Check sheet for the modelled part. Datum: model origin and axes. Units: mm. A direction names the side the tool comes from. Round coordinates to 2 decimals unless told otherwise and drop trailing zeros. Order: outer loops, then holes, each group sorted by start corner. A loop starts at its lowest first (then second) coordinate and runs counter-clockwise, first axis right, second up.
```python
from build123d import *

# Parameters (mm, degrees)
F2_R      = 31.4610783887
F2_R_2    = 24.995840748
F3_DEPTH  = 33.02
F4_R      = 38.1
F4_R_2    = 31.4610783887
F4_R_3    = 24.995840748
F5_DEPTH  = 35.56
F6_SIZE   = 12.7
F8_W      = 7.62
F8_H      = 11.43
F9_DEPTH  = 15.7618920784
F10_SIZE  = 5.08
F11_R     = 3.175
F12_DEPTH = 5.08
F13_R     = 3.175
F14_DEPTH = 5.08


with BuildPart() as f3:
    # F2 (on offset) → F3 (new body)
    with BuildSketch(Plane.XY.offset(-98.8788958639)):
        Circle(F2_R)
        Circle(F2_R_2, mode=Mode.SUBTRACT)
    extrude(amount=-F3_DEPTH)

    # F4 (on face) → F5 (join)
    with BuildSketch(Plane(origin=(0, 0, -131.8988958639), x_dir=(1, 0, 0), z_dir=(0, 0, -1))):
        Circle(F4_R)
        Circle(F4_R_2, mode=Mode.SUBTRACT)
        Circle(F4_R_2)
        Circle(F4_R_3, mode=Mode.SUBTRACT)
        Circle(F4_R_3)
    extrude(amount=F5_DEPTH)

    # F6
    f6_edges = [f3.edges().sort_by_distance(p)[0] for p in [
        (-38.1, 0, -167.458896),
    ]]
    chamfer(f6_edges, length=F6_SIZE)

    # F8 (on face) → F9 (join)
    with BuildSketch(Plane(origin=(0, 0, -167.4588958639), x_dir=(1, 0, 0), z_dir=(0, 0, -1))):
        with Locations((0, 29.3979875922)):
            Rectangle(F8_W, F8_H)
        Polygon((-12.3045016564, 20.5912418344), (-19.6515640351, 29.3471298192), (-25.4888226916, 24.4490882334), (-18.1417603129, 15.6932002486), align=None)
        Polygon((-22.6615902384, 7.8646251761), (-33.9179428553, 9.8494238468), (-35.2411419691, 2.3451887689), (-23.9847893522, 0.3603900981), align=None)
        Polygon((-22.4150688924, -8.5419370077), (-32.3137392576, -14.2569370077), (-28.5037392576, -20.8560505845), (-18.6050688924, -15.1410505845), align=None)
        Polygon((-11.6802876959, -20.9516319325), (-15.5895779341, -31.6923185881), (-8.4291201637, -34.2985120802), (-4.5198299255, -23.5578254246), align=None)
        Polygon((4.5198299255, -23.5578254246), (8.4291201637, -34.2985120802), (15.5895779341, -31.6923185881), (11.6802876959, -20.9516319325), align=None)
        Polygon((18.6050688924, -15.1410505845), (28.5037392576, -20.8560505845), (32.3137392576, -14.2569370077), (22.4150688924, -8.5419370077), align=None)
        Polygon((23.9847893522, 0.3603900981), (35.2411419691, 2.3451887689), (33.9179428553, 9.8494238468), (22.6615902384, 7.8646251761), align=None)
        Polygon((18.1417603129, 15.6932002486), (25.4888226916, 24.4490882334), (19.6515640351, 29.3471298192), (12.3045016564, 20.5912418344), align=None)
    extrude(amount=-F9_DEPTH)

    # F10
    f10_edges = [f3.edges().sort_by_distance(p)[0] for p in [
        (-34.579542, -6.097306, -167.458896),
        (-22.570193, -26.898109, -167.458896),
        (0, -35.112988, -167.458896),
        (22.570193, -26.898109, -167.458896),
        (34.579542, -6.097306, -167.458896),
        (30.408739, 17.556494, -167.458896),
        (12.009349, 32.995415, -167.458896),
        (-12.009349, 32.995415, -167.458896),
        (-30.408739, 17.556494, -167.458896),
    ]]
    chamfer(f10_edges, length=F10_SIZE)

    # F11 (on Right) → F12 (join)
    with BuildSketch(Plane.YZ):
        with BuildLine():
            Line((-5.6298612599, -163.2592975991), (-5.6298612599, -171.5561002624))
            ThreePointArc((-5.6298612599, -171.5561002624), (0.0380569816, -178.2537691491), (5.6162731016, -171.4812090256))
            Line((5.6162731016, -171.4812090256), (5.6162731016, -163.2592975991))
            Line((5.6162731016, -163.2592975991), (-5.6298612599, -163.2592975991))
        make_face()
        with Locations((0, -172.5388958639)):
            Circle(F11_R, mode=Mode.SUBTRACT)
    extrude(amount=F12_DEPTH)

    # F13 (on face) → F14 (join)
    with BuildSketch(Plane.YZ):
        with BuildLine():
            Line((-5.6212010458, -163.5551446258), (-5.6212010458, -171.4558557956))
            ThreePointArc((-5.6212010458, -171.4558557956), (-5.6255780847, -171.4788259602), (-5.6298612599, -171.5018138123))
            Line((-5.6298612599, -171.5018138123), (-5.6298612599, -171.5561002624))
            ThreePointArc((-5.6298612599, -171.5561002624), (0.0380569816, -178.2537691491), (5.6162731016, -171.4812090256))
            Line((5.6162731016, -171.4812090256), (5.6162731016, -163.5551446258))
            Line((5.6162731016, -163.5551446258), (-5.6212010458, -163.5551446258))
        make_face()
        with Locations((0, -172.5388958639)):
            Circle(F13_R, mode=Mode.SUBTRACT)
    extrude(amount=-F14_DEPTH)


solid = f3.part
```
Item 1: Go/stop test with flat-tipped pins: P1, Ø12, axis at x = -28, z = -155.5, coming from the -Y side; P2, Ø8, axis at y = 6, z = -150, coming from the +X side; P3, Ø12, axis at y = 1, z = -174, coming from the +X side. Record where each tip stops, or that it passes through.
Answer:
P1: stops at y = -31.07
P2: stops at x = 38.05
P3: stops at x = 5.08
Item 2: Release check for a two-part mould opening along X. For faces 5 (the cylindrical face through (-5.42, -24.4, -115.16)), 6 (the flat face through (28.213, 16.35, -164.883)), 7 (the flat face through (-34.57, -6.15, -159.99)) record: released by +X, released by -X, zero draft, split by the parting line, or undercut.
Answer:
face 5: undercut
face 6: released by +X
face 7: released by -X
Item 3: Sectioned sample at A-A (z = -130.5). Record the cut outline in (x, y), and give its area (3 significant figures).
Answer:
outline: circle Ø62.92 at (0, 0); hole circle Ø49.99 at (0, 0)
area: 1,150 mm2
Item 4: Scan lines: line 1 along Y through (x, z) = (0, -112); line 2 along Z through (x, y) = (-0.75, 0); line 3 along X through (y, z) = (2, -120.5). Record each from-to range of solid material in increasing order.
Answer:
line 1: y = -31.46 to -25, 25 to 31.46
line 2: z = -178.25 to -175.71, -169.36 to -131.9
line 3: x = -31.4 to -24.92, 24.92 to 31.4
Item 5: Access from +Z, -Z, +X, -X, +Y, -Y to the whole of each face (thin tool, end or side, straight path). Record for faces 1 (the flat face through (25.116, 18.9, -163.625)), 2 (the flat face through (-5.08, 0, -169)), 3 (the flat face through (34.59, -6.04, -159.99)), 4 (the flat face through (30.157, -9.186, -163.671)).
Answer:
face 1: -Z, +Y
face 2: -Z, -X, +Y, -Y
face 3: -Z, +X, -Y
face 4: -Z, -Y
